```python
from build123d import *

# Parameters (mm, degrees)
SKETCH1_W                      = 177.8
SKETCH1_H                      = 35.749524071
BOSS_EXTRUDE1_DEPTH            = 15.24
SKETCH2_W                      = 177.8
SKETCH2_H                      = 107.315000048
BOSS_EXTRUDE2_DEPTH            = 6.222024
CHAMFER1_SIZE                  = 12.7
F_8_0_199_DIAMETER_HOLE2_D     = 5.0546
CUT_EXTRUDE1_DEPTH             = 82.280000048
SKETCH8_W                      = 177.8
SKETCH8_H                      = 29.5275
BOSS_EXTRUDE3_DEPTH            = 66.04
SKETCH9_W                      = 152.4
SKETCH9_H                      = 12.7
CUT_EXTRUDE2_DEPTH             = 36.749524071
SKETCH10_W                     = 177.8
SKETCH10_H                     = 3.175
CUT_EXTRUDE3_DEPTH             = 108.315000048
SKETCH11_W                     = 13.208
SKETCH11_H                     = 8.255
CUT_EXTRUDE4_DEPTH             = 178.8
SKETCH12_W                     = 120.65
SKETCH12_H                     = 11.58875
CUT_EXTRUDE5_DEPTH             = 95.615000048
BOSS_EXTRUDE4_DEPTH            = 68.58
CHAMFER2_SIZE                  = 3.175
F_8_0_199_DIAMETER_HOLE1_D     = 5.0546
F_8_0_199_DIAMETER_HOLE1_DEPTH = 11.460774071
F_8_PLASTIC_INSERT_AT_2_COUNT  = 2
F_8_PLASTIC_INSERT_AT_2_PITCH  = 50.8


with BuildPart() as part:
    # Sketch1 → Boss-Extrude1 (new body)
    with BuildSketch(Plane.XY):
        with Locations((0, 59.912737965)):
            Rectangle(SKETCH1_W, SKETCH1_H)
    extrude(amount=BOSS_EXTRUDE1_DEPTH)

    # Sketch2 → Boss-Extrude2 (add)
    with BuildSketch(Plane.XZ.offset(-42.037975929)):
        with Locations((0, -12.382499976)):
            Rectangle(SKETCH2_W, SKETCH2_H)
    extrude(amount=-BOSS_EXTRUDE2_DEPTH)

    # Chamfer1
    chamfer1_edges = [part.edges().sort_by_distance(p)[0] for p in [
        (88.9, 45.148987929, 41.275000048),
        (-88.9, 45.148987929, 41.275000048),
    ]]
    chamfer(chamfer1_edges, length=CHAMFER1_SIZE)

    # #8 (0.199) Diameter Hole2 (through all)
    with Locations(Plane(origin=(0, 42.037975929, 0), x_dir=(-1, 0, 0), z_dir=(0, -1, 0))):
        with Locations((-44.45, -28.575000048), (0, -28.575000048), (44.45, -28.575000048)):
            Hole(F_8_0_199_DIAMETER_HOLE2_D / 2)

    # Sketch7 → Cut-Extrude1 (cut, through all)
    with BuildSketch(Plane.XY.offset(15.240000048)):
        with BuildLine():
            Line((-50.8, 72.54875), (50.8, 72.54875))
            ThreePointArc((50.8, 72.54875), (60.325, 63.02375), (50.8, 53.49875))
            Line((50.8, 53.49875), (-50.8, 53.49875))
            ThreePointArc((-50.8, 53.49875), (-60.325, 63.02375), (-50.8, 72.54875))
        make_face()
    extrude(amount=-CUT_EXTRUDE1_DEPTH, mode=Mode.SUBTRACT)

    # Sketch8 → Boss-Extrude3 (add)
    with BuildSketch(Plane(origin=(0, 0, 0), x_dir=(-1, 0, 0), z_dir=(0, 0, -1))):
        with Locations((0, 63.02375)):
            Rectangle(SKETCH8_W, SKETCH8_H)
        with BuildLine():
            Line((50.8, 72.54875), (-50.8, 72.54875))
            ThreePointArc((-50.8, 72.54875), (-60.325, 63.02375), (-50.8, 53.49875))
            Line((-50.8, 53.49875), (50.8, 53.49875))
            ThreePointArc((50.8, 53.49875), (60.325, 63.02375), (50.8, 72.54875))
        make_face(mode=Mode.SUBTRACT)
    extrude(amount=BOSS_EXTRUDE3_DEPTH)

    # Sketch9 → Cut-Extrude2 (cut, through all)
    with BuildSketch(Plane.XZ.offset(-42.037975929)):
        with Locations((0, -59.69)):
            Rectangle(SKETCH9_W, SKETCH9_H)
    extrude(amount=-CUT_EXTRUDE2_DEPTH, mode=Mode.SUBTRACT)

    # Sketch10 → Cut-Extrude3 (cut, through all)
    with BuildSketch(Plane(origin=(0, 0, -66.04), x_dir=(-1, 0, 0), z_dir=(0, 0, -1))):
        with Locations((0, 76.2)):
            Rectangle(SKETCH10_W, SKETCH10_H)
    extrude(amount=-CUT_EXTRUDE3_DEPTH, mode=Mode.SUBTRACT)

    # Sketch11 → Cut-Extrude4 (cut, through all)
    with BuildSketch(Plane(origin=(88.9, 0, 0), x_dir=(0, 0, -1), z_dir=(1, 0, 0))):
        with Locations((-8.636000048, 70.485)):
            Rectangle(SKETCH11_W, SKETCH11_H)
    extrude(amount=-CUT_EXTRUDE4_DEPTH, mode=Mode.SUBTRACT)

    # Sketch12 → Cut-Extrude5 (cut, through all)
    with BuildSketch(Plane(origin=(0, 0, -53.34), x_dir=(-1, 0, 0), z_dir=(0, 0, -1))):
        with Locations((0, 68.818125)):
            Rectangle(SKETCH12_W, SKETCH12_H)
    extrude(amount=-CUT_EXTRUDE5_DEPTH, mode=Mode.SUBTRACT)

    # Sketch13 → Boss-Extrude4 (add)
    with BuildSketch(Plane.XY.offset(15.240000048)):
        with BuildLine():
            Line((60.325, 63.02375), (50.8, 53.49875))
            ThreePointArc((50.8, 53.49875), (57.535192091, 56.288557909), (60.325, 63.02375))
        make_face()
        with BuildLine():
            Line((-60.325, 63.02375), (-50.8, 53.49875))
            ThreePointArc((-50.8, 53.49875), (-57.535192091, 56.288557909), (-60.325, 63.02375))
        make_face()
    extrude(amount=-BOSS_EXTRUDE4_DEPTH)

    # Chamfer2
    chamfer2_edges = [part.edges().sort_by_distance(p)[0] for p in [
        (-76.2, 58.325237965, -53.34),
        (76.2, 58.325237965, -53.34),
    ]]
    chamfer(chamfer2_edges, length=CHAMFER2_SIZE)

    # #8 (0.199) Diameter Hole1
    with Locations(Plane(origin=(9.884621419, 42.037975929, -19.494996768), x_dir=(-1, 0, 0), z_dir=(0, -1, 0))):
        with Locations((-15.515378581, -0.444996793), (35.284621419, -0.444996793)):
            Hole(F_8_0_199_DIAMETER_HOLE1_D / 2, depth=F_8_0_199_DIAMETER_HOLE1_DEPTH)

    # Sketch51 → #8 Plastic Insert (revolve, cut)
    with BuildSketch(Plane(origin=(25.4, 42.037975929, -19.049999976), x_dir=(0, 0, -1), z_dir=(1, 0, 0))):
        Polygon((0, 0), (0, 4.699), (2.8702, 4.699), (2.9972, 0), align=None)
    f_8_plastic_insert = revolve(axis=Axis((25.4, 152.037975929, -19.049999976), (0, -1, 0)), mode=Mode.SUBTRACT)

    # #8 Plastic Insert at 2: #8 Plastic Insert ×2
    with Locations(*[(-i * F_8_PLASTIC_INSERT_AT_2_PITCH, 0, 0) for i in range(1, F_8_PLASTIC_INSERT_AT_2_COUNT)]):
        add(f_8_plastic_insert, mode=Mode.SUBTRACT)


solid = part.part
```
Part model, mm, in its own coordinate system. A direction names the side the tool comes from. Round coordinates to 2 decimals unless told otherwise and drop trailing zeros. Write each loop counter-clockwise with the first axis right and the second up, starting at its lowest first coordinate (ties: lowest second). Pieces come first, ordered by that corner, then holes. Notation, with made-up numbers: (-39.75, -26.75) -> (2.25, -26.75) arc R21 ccw to (2.25, -9.75) -> close; hole circle Ø10 at (38, 31.25). An arc over 180 degrees is marked (long way). Return JSON: item names as keys, results as strings. Group by question number.
Q1. Saw through at C-C on x = -44.45. Write the cut outline in (y, z) (3 decimals).
Q2. Pin check, flat tips, straight feed: pin 1 (1 mm diameter, centred on x = 16.5, z = -36.5, fed in from +Y); pin 2 (6.5 mm diameter, centred on x = -69, y = 72.5, fed in from +Z); pin 3 (8 mm diameter, centred on x = -31, z = 24.5, fed in from +Y). Stop position of each tip, or through.
Q3. Probe L1, parallel to Z at x = -44.45, y = 46 (3 decimals); L2, parallel to Z at x = 25, y = 49; L3, parallel to X at y = 67, z = -13 (3 decimals). List the from-to ranges inside material, lowest first. Write a range as [from, to].
Q4. Mould opens along Z. For faces 6 (the flat face through (-82.461, 45.105, 35.014)), 7 (the cylindrical face through (27.81, 50.17, -19.81)), 8 (the flat face through (-76.2, 58, -61)) say: pulls with the +Z half, pulls with the -Z half, needs draft (parallel to the pull), parting line crosses it, or undercut.
Q5. Saw through at B-B on y = 71.5. Write the cut outline in (x, z) (3 decimals), plus the area to 3 significant figures.
Q6. Which spindle directions (+Z, -Z, +X, -X, +Y, -Y) get a long thin tool onto all of the face, cutting with end or side? Do faces 1 (the flat face through (-60.325, 69, -27)), 2 (the flat face through (-1, 51, -53.34)), 3 (the flat face through (-1, 45, 41.275)), 4 (the flat face through (75, 70, 2.032)), 5 (the conical face through (26.28, 44.35, -21.85)). Say none if no direction does.
Q7. Saw through at D-D on y = 50. Write the cut outline in (x, z) (3 decimals).
Q8. Saw through at A-A on z = -19.05. State how many separate pieces and enclosed holes the cut face has, plus the area to 3 significant figures.
Answer:
{
 "1": {"outline": "(42.038, -53.34) -> (53.499, -53.34) -> (53.499, 15.24) -> (48.26, 15.24) -> (48.26, 26.048) -> (42.038, 26.048) -> close; (42.038, 31.102) -> (48.26, 31.102) -> (48.26, 41.275) -> (42.038, 41.275) -> close"},
 "2": {"pin 1": "y = 53.5", "pin 2": "z = 2.03", "pin 3": "y = 48.26"},
 "3": {"L1": "[-53.34, 26.048], [31.102, 41.275]", "L2": "[-53.34, -21.55], [-16.55, 15.24]", "L3": "[-88.9, -60.325], [60.325, 88.9]"},
 "4": {"face 6": "pulls with the +Z half", "face 7": "undercut", "face 8": "needs draft"},
 "5": {"outline": "(-88.9, -66.04) -> (-76.2, -66.04) -> (-76.2, -56.515) -> (-73.025, -53.34) -> (-60.325, -53.34) -> (-60.325, 2.032) -> (-88.9, 2.032) -> close; (60.325, -53.34) -> (73.025, -53.34) -> (76.2, -56.515) -> (76.2, -66.04) -> (88.9, -66.04) -> (88.9, 2.032) -> (60.325, 2.032) -> close", "area": "3,500 mm2"},
 "6": {"face 1": "+Z, -Z, +Y", "face 2": "-Z, +Y, -Y", "face 3": "+Z, +X, -X, +Y, -Y", "face 4": "+Z, +X, -X, +Y", "face 5": "-Y"},
 "7": {"outline": "(-88.9, -66.04) -> (-76.2, -66.04) -> (-76.2, -56.515) -> (-73.025, -53.34) -> (73.025, -53.34) -> (76.2, -56.515) -> (76.2, -66.04) -> (88.9, -66.04) -> (88.9, 15.24) -> (-88.9, 15.24) -> close; hole circle Ø5.055 at (-25.4, -19.05); hole circle Ø5.055 at (25.4, -19.05)"},
 "8": {"separate pieces": "3", "enclosed holes": "0", "area": "3,210 mm2"}
}
